```python
from build123d import *

# Parameters (mm, degrees)
SKETCH1_W           = 165
SKETCH1_H           = 60
BOSS_EXTRUDE1_DEPTH = 10
SKETCH2_W           = 3.81
SKETCH2_H           = 5
CUT_EXTRUDE1_DEPTH  = 7.5
FILLET1_R           = 2.54


with BuildPart() as part:
    # Sketch1 → Boss-Extrude1 (new body)
    with BuildSketch(Plane(origin=(0, 0, 0), x_dir=(1, 0, 0), z_dir=(0, 1, 0))):
        Rectangle(SKETCH1_W, SKETCH1_H)
        Polygon((-75.04, 20.262432489), (-75.04, -20.262432489), (-12.226459283, 0), align=None, mode=Mode.SUBTRACT)
        Polygon((57.460458264, 22.165834991), (-57.834623171, 22.165834991), (-0.187082453, 3.569854115), align=None, mode=Mode.SUBTRACT)
        Polygon((74.852917547, 20.262432489), (74.852917547, -20.262432489), (12.039376829, 0), align=None, mode=Mode.SUBTRACT)
        Polygon((-57.834623171, -22.165834991), (-0.187082453, -3.569854115), (57.460458264, -22.165834991), align=None, mode=Mode.SUBTRACT)
    extrude(amount=BOSS_EXTRUDE1_DEPTH)

    # Sketch2 → Cut-Extrude1 (cut)
    with BuildSketch(Plane.ZY.offset(82.5)):
        with Locations((-12.7, 7.5)):
            Rectangle(SKETCH2_W, SKETCH2_H)
        with Locations((12.7, 7.5)):
            Rectangle(SKETCH2_W, SKETCH2_H)
    cut_extrude1 = extrude(amount=-CUT_EXTRUDE1_DEPTH, mode=Mode.SUBTRACT)

    # Mirror1: Cut-Extrude1 across plane
    add(cut_extrude1.mirror(Plane(origin=(0, 0, 0), x_dir=(0, 0, 1), z_dir=(1, 0, 0))), mode=Mode.SUBTRACT)

    # Fillet1
    fillet1_edges = [part.edges().sort_by_distance(p)[0] for p in [
        (0, 10, -30),
        (0, 10, 30),
    ]]
    fillet(fillet1_edges, radius=FILLET1_R)


solid = part.part
```
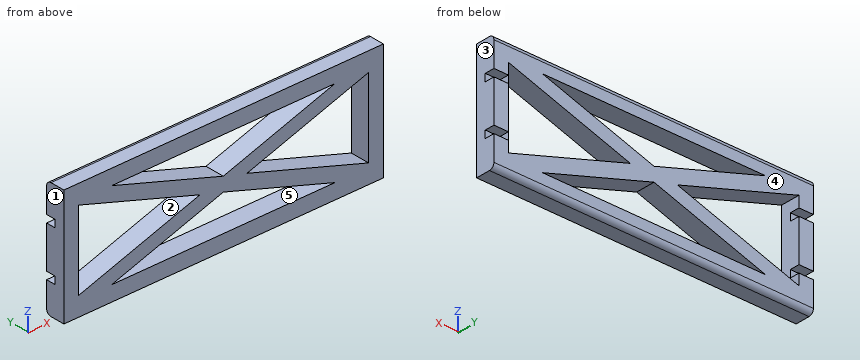
Input: part model. Units: mm. Frame: model coordinates. Face numbers are marked on the shaded views. A direction names the side the tool comes from. Give positions to 0.01 mm unless a question says otherwise; leave off trailing zeros. Order: outer loops, then holes, each group sorted by start corner. A loop starts at its lowest first (then second) coordinate and runs counter-clockwise, first axis right, second up.
1. Line query: probe 1 along Z at (x, y) = (-15, 3.5); probe 2 along Z at (x, y) = (-75, 0.75); probe 3 along Z at (x, y) = (26, 6). Output: solid intervals per line, ascending.
Computed:
probe 1: z = -30 to -22.17, -8.35 to -0.89, 0.89 to 8.35, 22.17 to 30
probe 2: z = -30 to -20.25, 20.25 to 30
probe 3: z = -30 to -22.17, -12.02 to -4.5, 4.5 to 12.02, 22.17 to 30
2. Cut plane A-A (y = 1.5). Return loops of the section in (x, z).
Computed:
outline: (-82.5, -30) - (82.5, -30) - (82.5, 30) - (-82.5, 30) - close; hole (-75.04, -20.26) - (-12.23, 0) - (-75.04, 20.26) - close; hole (-57.83, -22.17) - (57.46, -22.17) - (-0.19, -3.57) - close; hole (-57.83, 22.17) - (-0.19, 3.57) - (57.46, 22.17) - close; hole (12.04, 0) - (74.85, -20.26) - (74.85, 20.26) - close
3. Cut plane C-C (z = 1.5). Return loops of the section in (x, y), and give its area (3 significant figures).
Computed:
outline: (-82.5, 0) - (-75.04, 0) - (-75.04, 10) - (-82.5, 10) - close; (-16.88, 0) - (16.69, 0) - (16.69, 10) - (-16.88, 10) - close; (74.85, 0) - (82.5, 0) - (82.5, 10) - (74.85, 10) - close
area: 487 mm2
4. Pin query (flat end, axial travel): pin 1 Ø1.9 at (y, z) = (6.5, 12) entering from +X; pin 2 Ø1.9 at (x, z) = (79.5, -13) entering from +Y. Return the tip coordinate at first contact, or that it passes through.
Computed:
pin 1: stops at x = 75
pin 2: stops at y = 5
5. Draft query along X for the marked faces 3, 4 and 5. Return one class per face: released by +X, released by -X, zero draft, split by the parting line, or undercut.
Computed:
face 3: released by +X
face 4: zero draft
face 5: undercut
6. Set-up query: the marked faces 1 and 2. Return all of +Z, -Z, +X, -X, +Y, -Y with unobstructed straight access to the full face (end or side cutting, diameter ignored); none if empty.
Computed:
face 1: +Z, -Z, -X, +Y, -Y
face 2: +Y, -Y
7. Cut plane D-D (x = 52.5). Return loops of the section in (y, z), and give its area (3 significant figures).
Computed:
outline: (0, -30) - (7.46, -30) arc R2.54 ccw to (10, -27.46) - (10, -22.17) - (0, -22.17) - close; (0, -20.57) - (10, -20.57) - (10, -13.05) - (0, -13.05) - close; (0, 13.05) - (10, 13.05) - (10, 20.57) - (0, 20.57) - close; (0, 22.17) - (10, 22.17) - (10, 27.46) arc R2.54 ccw to (7.46, 30) - (0, 30) - close
area: 304 mm2
8. Cut plane B-B (x = -5.5). Return loops of the section in (y, z), and give its area (3 significant figures).
Computed:
outline: (0, -30) - (7.46, -30) arc R2.54 ccw to (10, -27.46) - (10, -22.17) - (0, -22.17) - close; (0, -5.28) - (10, -5.28) - (10, 5.28) - (0, 5.28) - close; (0, 22.17) - (10, 22.17) - (10, 27.46) arc R2.54 ccw to (7.46, 30) - (0, 30) - close
area: 260 mm2
